Read the model definition and answer for the solid it produces. Units are mm, in the model's axes. Give positions to 0.01 mm unless a question says otherwise; leave off trailing zeros. Order: outer loops, then holes, each group sorted by start corner. A loop starts at its lowest first (then second) coordinate and runs counter-clockwise, first axis right, second up. Notation, with made-up numbers: M 39.25,37.25 L 86.25,37.25 A16 cw 86.25,61.25 Z; hole C 80,-29 d5. An arc over 180 degrees is marked long. One line per item, written item: value. Start each with the question number.
from build123d import *

# Parameters (mm, degrees)
F0_W     = 186.9
F0_H     = 111.2
F1_DEPTH = 10
F2_R     = 10
F3_SIZE  = 2
F4_R     = 6


with BuildPart() as f1:
    # F0 (on Top) → F1 (new body)
    with BuildSketch(Plane.XY):
        Rectangle(F0_W, F0_H)
    extrude(amount=F1_DEPTH)

    # F2
    f2_edges = [f1.edges().sort_by_distance(p)[0] for p in [
        (93.45, 55.6, 5),
        (93.45, -55.6, 5),
        (-93.45, 55.6, 5),
        (-93.45, -55.6, 5),
    ]]
    fillet(f2_edges, radius=F2_R)

    # F3
    f3_edges = [f1.edges().sort_by_distance(p)[0] for p in [
        (0, 55.6, 10),
    ]]
    chamfer(f3_edges, length=F3_SIZE)

    # F4
    f4_edges = [f1.edges().sort_by_distance(p)[0] for p in [
        (0, 55.6, 0),
    ]]
    fillet(f4_edges, radius=F4_R)


solid = f1.part
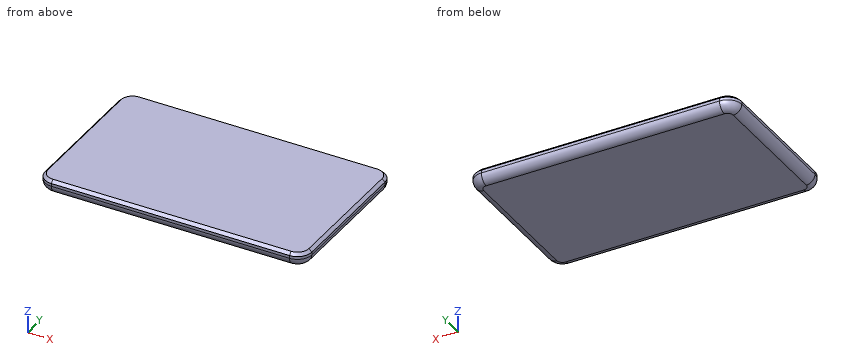
Q1. Find section A-A, the plane x = 24.5. Give the vertices of the cut face in (y, z), then the cut area to 3 significant figures.
Q2. Each of these flat-tipped pins is pushed along its axis until it touches: pin 1 (1 mm diameter, centred on x = -38, z = 2, fed in from -Y); pin 2 (4 mm diameter, centred on x = 24, z = 3.5, fed in from +Y); pin 3 (1.5 mm diameter, centred on y = 2.5, z = 1.5, fed in from +X). Where does it stop, or does it pass through?
Q3. Consider probe 1 along Y at (x, z) = (-44, 1.5); probe 2 along X at (y, z) = (-28, 5.75); probe 3 along Z at (x, y) = (30, -50). Determine where each line is inside the solid, lowest interval first.
Evaluation:
1. outline: M -55.6,6 A6 ccw -49.6,0 L 49.6,0 A6 ccw 55.6,6 L 55.6,8 L 53.6,10 L -53.6,10 L -55.6,8 Z
1. area: 1,090 mm2
2. pin 1: y = -54.47
2. pin 2: y = 55.58
2. pin 3: x = 92.13
3. probe 1: -53.57 to 53.57
3. probe 2: -93.44 to 93.44
3. probe 3: 0.01 to 10
